Read the model definition and answer for the solid it produces. Units are mm, in the model's axes. A direction names the side the tool comes from. Coordinates: 2 decimals unless noted, no trailing zeros. Loops run counter-clockwise (first coordinate to the right, second up) from the corner with the lowest first, then second, coordinate; pieces in that order, holes last.
Autodesk Inventor part; units mm, degrees
ref_plane "YZ Plane" through (0, 0, 0) normal (1, 0, 0) x (0, 1, 0)
ref_plane "XZ Plane" through (0, 0, 0) normal (0, 1, 0) x (-1, 0, 0)
ref_plane "XY Plane" through (0, 0, 0) normal (0, 0, 1) x (1, 0, 0)
sketch "Sketch1" plane through (0, 0, 0) normal (1, 0, 0) x (0, 1, 0)
  line L0 (0, 0) -> (21.59, 0)
  line L1 (21.59, 0) -> (21.59, -21.59)
  line L2 (21.59, -21.59) -> (0, -21.59)
  line L3 (0, -21.59) -> (0, 0)
  circle A0 centre (17.7098, -3.8802) radius 1.905
  circle A1 centre (17.7098, -17.7098) radius 1.905
  circle A2 centre (3.8802, -17.7098) radius 1.905
  circle A3 centre (3.8802, -3.8802) radius 1.905
  dimension "d0" = 21.59
  dimension "d1" = 21.59
  dimension "d3" = 3.81
  dimension "d4" = 3.81
  dimension "d5" = 3.81
  dimension "d6" = 3.81
extrude "Extrusion1" add sketch "Sketch1" along normal blind 2.54
sketch "Sketch2" plane through (2.54, 0, 0) normal (1, 0, 0) x (0, 0, -1)
  line L0 (21.59, 0) -> (21.59, 21.59)
  line L1 (21.59, 21.59) -> (0, 21.59)
  line L2 (0, 21.59) -> (0, 0)
  circle A0 centre (10.795, 10.795) radius 6.985
  dimension "d9" = 13.97
extrude "Extrusion2" cut sketch "Sketch2" against normal blind 1.27
sketch "Sketch3" plane through (1.27, 10.795, -10.795) normal (1, 0, 0) x (0, 0, -1)
  circle A0 centre (0, 0) radius 3.429
  point P0 (-10.795, -10.795)
  dimension "d12" = 6.858
extrude "Extrusion3" cut sketch "Sketch3" against normal blind 24.13
properties part number "BearingSpacer"
Q1. Flat-ended cylindrical pins translate along their axes: pin 1 Ø4 at (y, z) = (10.795, -10.795) entering from -X; pin 2 Ø4 at (y, z) = (13, -12) entering from +X; pin 3 Ø5 at (y, z) = (15.5, -4.5) entering from -X. Find the tip coordinate at first contact, or state that the pin passes through.
Findings below:
pin 1: passes through
pin 2: stops at x = 1.27
pin 3: stops at x = 0
Q2. A cutting plane is placed at D-D (z = -17.25). Give the vertices of the cut face in (x, y), then the cut area to 3 significant figures.
Findings below:
outline: (0, 0) - (2.54, 0) - (2.54, 2.03) - (0, 2.03) - close; (0, 5.73) - (2.54, 5.73) - (2.54, 8.13) - (1.27, 8.13) - (1.27, 13.46) - (2.54, 13.46) - (2.54, 15.86) - (0, 15.86) - close; (0, 19.56) - (2.54, 19.56) - (2.54, 21.59) - (0, 21.59) - close
area: 29.3 mm2
Q3. A cutting plane is placed at A-A (z = -12.25). Give the vertices of the cut face in (x, y).
Findings below:
outline: (0, 0) - (2.54, 0) - (2.54, 3.96) - (1.27, 3.96) - (1.27, 7.69) - (0, 7.69) - close; (0, 13.9) - (1.27, 13.9) - (1.27, 17.63) - (2.54, 17.63) - (2.54, 21.59) - (0, 21.59) - close
Q4. A cutting plane is placed at C-C (x = 0.4). Give the vertices of the cut face in (y, z) (3 decimals).
Findings below:
outline: (0, -21.59) - (21.59, -21.59) - (21.59, 0) - (0, 0) - close; hole circle Ø3.81 at (3.88, -17.71); hole circle Ø3.81 at (3.88, -3.88); hole circle Ø6.858 at (10.795, -10.795); hole circle Ø3.81 at (17.71, -17.71); hole circle Ø3.81 at (17.71, -3.88)
Q5. Straight lines are drawn through the part: probe 1 along Y at (x, z) = (0.75, -17.75); probe 2 along Z at (x, y) = (0.25, 3.75); probe 3 along Z at (x, y) = (1.2, 10.75). For each, find the intervals that lie inside material, in ascending order.
Findings below:
probe 1: y = 0 to 1.98, 5.78 to 15.81, 19.61 to 21.59
probe 2: z = -21.59 to -19.61, -15.81 to -5.78, -1.98 to 0
probe 3: z = -21.59 to -14.22, -7.37 to 0
Q6. A cutting plane is placed at B-B (y = 10.5). Give the vertices of the cut face in (x, z), then the cut area to 3 significant figures.
Findings below:
outline: (0, -21.59) - (2.54, -21.59) - (2.54, -17.77) - (1.27, -17.77) - (1.27, -14.21) - (0, -14.21) - close; (0, -7.38) - (1.27, -7.38) - (1.27, -3.82) - (2.54, -3.82) - (2.54, 0) - (0, 0) - close
area: 28.4 mm2
Q7. Determine the mould class of faces 1 (the face through (0, 8, -8)), 2 (the face through (1, 11, 0)), 3 (the face through (1.25, 4.9, -5.49)) for opening direction Z: +Z half, -Z half, draft (parallel to the pull), parting line (faces both ways), or undercut.
Findings below:
face 1: draft
face 2: +Z half
face 3: undercut
Q8. Which of the six approach directions +Z, -Z, +X, -X, +Y, -Y give full straight-line access (tool end or side, diameter ignored) to faces 4 (the face through (0.644, 14.195, -10.349)), 5 (the face through (1.27, 14, -9))?
Findings below:
face 4: +X, -X
face 5: +X
